from build123d import *

# Parameters (mm, degrees)
SKETCH_R     = 1
PAD_DEPTH    = 12
SKETCH002_W  = 11.430722
SKETCH002_H  = 8.057475
POCKET_DEPTH = 17


with BuildPart() as part:
    # Sketch → Pad (new body)
    with BuildSketch(Plane.YZ):
        with BuildLine():
            Line((0, 0), (17, 0))
            Line((17, 0), (17, 3))
            Line((17, 3), (4, 3))
            Line((4, 3), (4, 9.067998))
            ThreePointArc((4, 9.067998), (2, 11.067998), (0, 9.067998))
            Line((0, 9.067998), (0, 0))
        make_face()
        with Locations((2, 9.067998)):
            Circle(SKETCH_R, mode=Mode.SUBTRACT)
    extrude(amount=PAD_DEPTH)

    # Sketch002 (on Face2 of Pad) → Pocket (cut)
    with BuildSketch(Plane.ZX.offset(17)):
        with Locations((7.505266, 5.98249)):
            Rectangle(SKETCH002_W, SKETCH002_H)
    extrude(amount=-POCKET_DEPTH, mode=Mode.SUBTRACT)


solid = part.part
Work out the finished part from the listing and answer in its coordinate system (mm). A direction names the side the tool comes from. Round coordinates to 2 decimals unless told otherwise and drop trailing zeros. Write each loop counter-clockwise with the first axis right and the second up, starting at its lowest first coordinate (ties: lowest second). Pieces come first, ordered by that corner, then holes. Notation, with made-up numbers: (89.25, 87) -> (138.25, 87) arc R27 ccw to (138.25, 105) -> close; hole circle Ø3 at (77.5, 22.25). An arc over 180 degrees is marked (long way). Answer as CSV lines item,"result". Start each with the question number.
(1) The part is cut by section D-D, the plane y = 14.75. Give the vertices of the cut face in (x, z).
(2) The mould has two halves that part along Y. Classify faces 4 (the cylindrical face through (0.96, 1.26, 9.74)), 5 (the flat face through (10.011, 3.5, 4.3)), 6 (the cylindrical face through (10.99, 1.26, 9.74)), 7 (the flat face through (6, 17, 1)): +Y half, -Y half, draft (parallel to the pull), parting line (faces both ways), or undercut.
(3) The part is cut by section A-A, the plane z = 5. Give the vertices of the cut face in (x, y), then the cut area to 3 significant figures.
(4) Each of these flat-tipped pins is pushed along its axis until it touches: pin 1 (1.6 mm diameter, centred on x = 11.5, y = 11, fed in from +Z); pin 2 (3 mm diameter, centred on y = 6, z = 7.5, fed in from +X); pin 3 (2 mm diameter, centred on x = 0.5, z = 7, fed in from +Y). Where does it stop, or does it pass through?
(5) A tool of negligible diameter and unlimited length cuts with its end or side. For faces 1 (the flat face through (6, 9, 1.79)), 2 (the flat face through (12, 6, 2)), 3 (the flat face through (11, 11, 3)), from which of +Z, -Z, +X, -X, +Y, -Y can it reach the whole face along a straight path? Write none if from no direction.
(6) The part is cut by section B-B, the plane y = 2. Give the vertices of the cut face in (x, z), then the cut area to 3 significant figures.
(7) The part is cut by section C-C, the plane z = 9.5. Give the vertices of the cut face in (x, y), then the cut area to 3 significant figures.
(8) Find the intervals of material crossed by probe 1 along X at (y, z) = (10, 2); probe 2 along Z at (x, y) = (10.8, 2); probe 3 along Z at (x, y) = (10.75, 8.5), in increasing order.
Output values:
1,outline,"(0, 0) -> (12, 0) -> (12, 3) -> (10.01, 3) -> (10.01, 1.79) -> (1.95, 1.79) -> (1.95, 3) -> (0, 3) -> close"
2,face 4,"undercut"
2,face 5,"draft"
2,face 6,"undercut"
2,face 7,"+Y half"
3,outline,"(0, 0) -> (1.95, 0) -> (1.95, 4) -> (0, 4) -> close; (10.01, 0) -> (12, 0) -> (12, 4) -> (10.01, 4) -> close"
3,area,"15.8 mm²"
4,pin 1,"stops at z = 3"
4,pin 2,"passes through"
4,pin 3,"stops at y = 4"
5,face 1,"+Z, +Y, -Y"
5,face 2,"+Z, -Z, +X, +Y, -Y"
5,face 3,"+Z, +X, -X, +Y"
6,outline,"(0, 0) -> (12, 0) -> (12, 8.07) -> (10.01, 8.07) -> (10.01, 1.79) -> (1.95, 1.79) -> (1.95, 8.07) -> (0, 8.07) -> close; (0, 10.07) -> (1.95, 10.07) -> (1.95, 11.07) -> (0, 11.07) -> close; (10.01, 10.07) -> (12, 10.07) -> (12, 11.07) -> (10.01, 11.07) -> close"
6,area,"50.2 mm²"
7,outline,"(0, 0.05) -> (1.95, 0.05) -> (1.95, 1.1) -> (0, 1.1) -> close; (0, 2.9) -> (1.95, 2.9) -> (1.95, 3.95) -> (0, 3.95) -> close; (10.01, 0.05) -> (12, 0.05) -> (12, 1.1) -> (10.01, 1.1) -> close; (10.01, 2.9) -> (12, 2.9) -> (12, 3.95) -> (10.01, 3.95) -> close"
7,area,"8.29 mm²"
8,probe 1,"x = 0 to 1.95, 10.01 to 12"
8,probe 2,"z = 0 to 8.07, 10.07 to 11.07"
8,probe 3,"z = 0 to 3"
